```python
from build123d import *

# Parameters (mm, degrees)
SKETCH1_W            = 35
SKETCH1_H            = 30
SKETCH1_R            = 2.1
BOSS_EXTRUDE1_DEPTH  = 5
SKETCH2_W            = 30
SKETCH2_H            = 17
BOSS_EXTRUDE2_DEPTH  = 5
BOSS_EXTRUDE3_START  = -28
BOSS_EXTRUDE3_DEPTH  = 37
CUT_EXTRUDE1_REACH   = 66.542
CUT_EXTRUDE1_START   = -4.5
SKETCH5_W            = 36
SKETCH5_H            = 12.013565991
SKETCH6_W            = 2.1
SKETCH6_H            = 35.25
CUT_EXTRUDE2_DEPTH   = 5
SKETCH7_R            = 2.1
CUT_EXTRUDE3_DEPTH   = 17
SKETCH8_W            = 1.9
SKETCH8_H            = 19
SKETCH8_W_2          = 2.4
BOSS_EXTRUDE4_DEPTH  = 11
SKETCH9_W            = 9.9
SKETCH9_H            = 8
SKETCH9_W_2          = 7.5
BOSS_EXTRUDE5_DEPTH  = 5
BOSS_EXTRUDE6_DEPTH  = 2
BOSS_EXTRUDE7_START  = -13
SKETCH12_R           = 3.3
SKETCH12_R_2         = 2.1
BOSS_EXTRUDE7_DEPTH  = 1
BOSS_EXTRUDE8_START  = -23
SKETCH12_2_R         = 3.3
SKETCH12_2_R_2       = 2.1
BOSS_EXTRUDE8_DEPTH  = 1
SKETCH13_W           = 21.9
SKETCH13_H           = 19
BOSS_EXTRUDE9_DEPTH  = 2
SKETCH14_W           = 1.9
SKETCH14_H           = 19
BOSS_EXTRUDE10_DEPTH = 11
SKETCH15_W           = 21.9
SKETCH15_H           = 19
BOSS_EXTRUDE11_DEPTH = 2
CUT_EXTRUDE4_START   = -36
SKETCH16_R           = 2.1
CUT_EXTRUDE4_DEPTH   = 36
BOSS_EXTRUDE12_START = -2
SKETCH17_R           = 3.3
SKETCH17_R_2         = 2.1
BOSS_EXTRUDE12_DEPTH = 1
BOSS_EXTRUDE13_START = -12
SKETCH17_2_R         = 3.3
SKETCH17_2_R_2       = 2.1
BOSS_EXTRUDE13_DEPTH = 1
CUT_EXTRUDE5_REACH   = 74.341
SKETCH19_R           = 4.5
CUT_EXTRUDE6_REACH   = 69.181
SKETCH20_R           = 1.75
SKETCH21_R           = 1.6
CUT_EXTRUDE7_DEPTH   = 95.781405877


with BuildPart() as part:
    # Sketch1 → Boss-Extrude1 (new body)
    with BuildSketch(Plane(origin=(0, 0, 0), x_dir=(1, 0, 0), z_dir=(0, 1, 0))):
        Rectangle(SKETCH1_W, SKETCH1_H)
        with Locations(Location((12, 9, 0), (0, 0, 270))):
            Circle(SKETCH1_R, mode=Mode.SUBTRACT)
        with Locations(Location((12, -9, 0), (0, 0, 90))):
            Circle(SKETCH1_R, mode=Mode.SUBTRACT)
        with Locations(Location((-12, -9, 0), (0, 0, 270))):
            Circle(SKETCH1_R, mode=Mode.SUBTRACT)
        with Locations(Location((-12, 9, 0), (0, 0, 90))):
            Circle(SKETCH1_R, mode=Mode.SUBTRACT)
    extrude(amount=BOSS_EXTRUDE1_DEPTH)

    # Sketch2 → Boss-Extrude2 (add)
    with BuildSketch(Plane.ZY.offset(17.5)):
        with Locations((0, -3.5)):
            Rectangle(SKETCH2_W, SKETCH2_H)
    extrude(amount=BOSS_EXTRUDE2_DEPTH)

    # Sketch3 → Boss-Extrude3 (add)
    with BuildSketch(Plane(origin=(17.5, 0, 0), x_dir=(0, 0, -1), z_dir=(1, 0, 0)).offset(BOSS_EXTRUDE3_START)):
        with BuildLine():
            Line((-41, 0), (41, 0))
            Line((41, 0), (41, -12))
            Line((41, -12), (37.43, -12))
            Line((37.43, -12), (37.43, -18))
            Line((37.43, -18), (35.03, -18))
            Line((35.03, -18), (35.03, -12))
            Line((35.03, -12), (35.03, -10.095119046))
            ThreePointArc((35.03, -10.095119046), (34.83, -1.9), (34.63, -10.095119046))
            Line((34.63, -10.095119046), (34.63, -12))
            Line((34.63, -12), (34.63, -18))
            Line((34.63, -18), (32.23, -18))
            Line((32.23, -18), (32.23, -12))
            Line((32.23, -12), (-32.23, -12))
            Line((-32.23, -12), (-32.23, -18))
            Line((-32.23, -18), (-34.63, -18))
            Line((-34.63, -18), (-34.63, -12))
            Line((-34.63, -12), (-34.63, -10.095119046))
            ThreePointArc((-34.63, -10.095119046), (-34.83, -1.9), (-35.03, -10.095119046))
            Line((-35.03, -10.095119046), (-35.03, -12))
            Line((-35.03, -12), (-35.03, -18))
            Line((-35.03, -18), (-37.43, -18))
            Line((-37.43, -18), (-37.43, -12))
            Line((-37.43, -12), (-41, -12))
            Line((-41, -12), (-41, 0))
        make_face()
    extrude(amount=-BOSS_EXTRUDE3_DEPTH)

    # Sketch5 → Cut-Extrude1 (cut, up to next)
    with BuildSketch(Plane.ZY.offset(22.5).offset(CUT_EXTRUDE1_START), mode=Mode.PRIVATE) as cut_extrude1_sk1:
        with Locations((0, -5.993217004)):
            Rectangle(SKETCH5_W, SKETCH5_H)
    cut_extrude1_tool1 = extrude(cut_extrude1_sk1.sketch, amount=-CUT_EXTRUDE1_REACH, mode=Mode.PRIVATE) & part.part
    add(cut_extrude1_tool1.solids().sort_by_distance((-18, -5.993217, 0))[0], mode=Mode.SUBTRACT)

    # Sketch6 → Cut-Extrude2 (cut)
    with BuildSketch(Plane(origin=(0, 5, 0), x_dir=(1, 0, 0), z_dir=(0, 1, 0))):
        with Locations((-21.45, -2.625)):
            Rectangle(SKETCH6_W, SKETCH6_H)
    extrude(amount=-CUT_EXTRUDE2_DEPTH, mode=Mode.SUBTRACT)

    # Sketch7 → Cut-Extrude3 (cut)
    with BuildSketch(Plane(origin=(0, 5, 0), x_dir=(1, 0, 0), z_dir=(0, 1, 0))):
        with Locations(Location((-29.9, -20.25, 0), (0, 0, 270))):
            Circle(SKETCH7_R)
        with Locations(Location((-41.9, 20.25, 0), (0, 0, 270))):
            Circle(SKETCH7_R)
    extrude(amount=-CUT_EXTRUDE3_DEPTH, mode=Mode.SUBTRACT)

    # Sketch8 → Boss-Extrude4 (add)
    with BuildSketch(Plane(origin=(0, 0, 0), x_dir=(1, 0, 0), z_dir=(0, 1, 0))):
        with BuildLine():
            Line((-47.5, 10.25), (-34.9, 10.25))
            ThreePointArc((-34.9, 10.25), (-32.778679656, 11.128679656), (-31.9, 13.25))
            Line((-31.9, 13.25), (-31.9, 26.051552427))
            Line((-31.9, 26.051552427), (-30.3, 26.051552427))
            Line((-30.3, 26.051552427), (-30.3, 11.65))
            ThreePointArc((-30.3, 11.65), (-31.178679656, 9.528679656), (-33.3, 8.65))
            Line((-33.3, 8.65), (-47.5, 8.65))
            Line((-47.5, 8.65), (-47.5, 10.25))
        make_face()
        with Locations((-18.95, -20.25)):
            Rectangle(SKETCH8_W, SKETCH8_H)
        with Locations((-38.7, -20.25)):
            Rectangle(SKETCH8_W_2, SKETCH8_H)
    extrude(amount=BOSS_EXTRUDE4_DEPTH)

    # Sketch9 → Boss-Extrude5 (add)
    with BuildSketch(Plane(origin=(0, 0, 0), x_dir=(1, 0, 0), z_dir=(0, 1, 0))):
        with Locations((-15.45, 19)):
            Rectangle(SKETCH9_W, SKETCH9_H)
        with Locations((-14.25, -19)):
            Rectangle(SKETCH9_W_2, SKETCH9_H)
    extrude(amount=BOSS_EXTRUDE5_DEPTH)

    # Sketch10 → Boss-Extrude6 (add)
    with BuildSketch(Plane(origin=(0, 11, 0), x_dir=(1, 0, 0), z_dir=(0, 1, 0))):
        with BuildLine():
            Line((-30.3, 26.051552427), (-47.5, 26.051552427))
            Line((-47.5, 26.051552427), (-47.5, 8.65))
            Line((-47.5, 8.65), (-33.3, 8.65))
            ThreePointArc((-33.3, 8.65), (-31.178679656, 9.528679656), (-30.3, 11.65))
            Line((-30.3, 11.65), (-30.3, 26.051552427))
        make_face()
    extrude(amount=BOSS_EXTRUDE6_DEPTH)

    # Sketch12 → Boss-Extrude7 (add)
    with BuildSketch(Plane.XZ.offset(12).offset(BOSS_EXTRUDE7_START)):
        with Locations(Location((-41.9, -20.25, 0), (0, 0, 270))):
            Circle(SKETCH12_R)
        with Locations(Location((-41.9, -20.25, 0), (0, 0, 90))):
            Circle(SKETCH12_R_2, mode=Mode.SUBTRACT)
    extrude(amount=BOSS_EXTRUDE7_DEPTH)

    # Sketch12<2> → Boss-Extrude8 (add)
    with BuildSketch(Plane.XZ.offset(12).offset(BOSS_EXTRUDE8_START)):
        with Locations(Location((-41.9, -20.25, 0), (0, 0, 270))):
            Circle(SKETCH12_2_R)
        with Locations(Location((-41.9, -20.25, 0), (0, 0, 90))):
            Circle(SKETCH12_2_R_2, mode=Mode.SUBTRACT)
    extrude(amount=BOSS_EXTRUDE8_DEPTH)

    # Sketch13 → Boss-Extrude9 (add)
    with BuildSketch(Plane(origin=(0, 11, 0), x_dir=(1, 0, 0), z_dir=(0, 1, 0))):
        with Locations((-28.95, -20.25)):
            Rectangle(SKETCH13_W, SKETCH13_H)
    extrude(amount=-BOSS_EXTRUDE9_DEPTH)

    # Sketch14 → Boss-Extrude10 (add)
    with BuildSketch(Plane(origin=(0, 11, 0), x_dir=(1, 0, 0), z_dir=(0, 1, 0))):
        with Locations((-18.95, -20.25)):
            Rectangle(SKETCH14_W, SKETCH14_H)
    extrude(amount=BOSS_EXTRUDE10_DEPTH)

    # Sketch15 → Boss-Extrude11 (add)
    with BuildSketch(Plane(origin=(0, 22, 0), x_dir=(1, 0, 0), z_dir=(0, 1, 0))):
        with Locations((-28.95, -20.25)):
            Rectangle(SKETCH15_W, SKETCH15_H)
    extrude(amount=BOSS_EXTRUDE11_DEPTH)

    # Sketch16 → Cut-Extrude4 (cut)
    with BuildSketch(Plane.XZ.offset(12).offset(CUT_EXTRUDE4_START)):
        with Locations(Location((-29.9, 20.25, 0), (0, 0, 90))):
            Circle(SKETCH16_R)
        with Locations(Location((-41.9, -20.25, 0), (0, 0, 90))):
            Circle(SKETCH16_R)
    extrude(amount=CUT_EXTRUDE4_DEPTH, mode=Mode.SUBTRACT)

    # Sketch17 → Boss-Extrude12 (add)
    with BuildSketch(Plane(origin=(0, 24, 0), x_dir=(1, 0, 0), z_dir=(0, 1, 0)).offset(BOSS_EXTRUDE12_START)):
        with Locations(Location((-29.9, -20.25, 0), (0, 0, 270))):
            Circle(SKETCH17_R)
        with Locations(Location((-29.9, -20.25, 0), (0, 0, 270))):
            Circle(SKETCH17_R_2, mode=Mode.SUBTRACT)
    extrude(amount=-BOSS_EXTRUDE12_DEPTH)

    # Sketch17<2> → Boss-Extrude13 (add)
    with BuildSketch(Plane(origin=(0, 24, 0), x_dir=(1, 0, 0), z_dir=(0, 1, 0)).offset(BOSS_EXTRUDE13_START)):
        with Locations(Location((-29.9, -20.25, 0), (0, 0, 270))):
            Circle(SKETCH17_2_R)
        with Locations(Location((-29.9, -20.25, 0), (0, 0, 270))):
            Circle(SKETCH17_2_R_2, mode=Mode.SUBTRACT)
    extrude(amount=-BOSS_EXTRUDE13_DEPTH)

    # Sketch19 → Cut-Extrude5 (cut, up to next)
    with BuildSketch(Plane.XZ.offset(12), mode=Mode.PRIVATE) as cut_extrude5_sk1:
        with Locations(Location((-29.9, 20.25, 0), (0, 0, 270))):
            Circle(SKETCH19_R)
    cut_extrude5_tool1 = extrude(cut_extrude5_sk1.sketch, amount=-CUT_EXTRUDE5_REACH, mode=Mode.PRIVATE) & part.part
    add(cut_extrude5_tool1.solids().sort_by_distance((-29.9, -12, 20.25))[0], mode=Mode.SUBTRACT)

    # Sketch20 → Cut-Extrude6 (cut, up to next)
    with BuildSketch(Plane(origin=(0, 0, 0), x_dir=(1, 0, 0), z_dir=(0, 1, 0)), mode=Mode.PRIVATE) as cut_extrude6_sk1:
        with Locations(Location((-34.5, 4.15, 0), (0, 0, 270))):
            Circle(SKETCH20_R)
    cut_extrude6_tool1 = extrude(cut_extrude6_sk1.sketch, amount=-CUT_EXTRUDE6_REACH, mode=Mode.PRIVATE) & part.part
    # Sketch20 → Cut-Extrude6 (cut, up to next)
    with BuildSketch(Plane(origin=(0, 0, 0), x_dir=(1, 0, 0), z_dir=(0, 1, 0)), mode=Mode.PRIVATE) as cut_extrude6_sk2:
        with Locations(Location((-44.5, -17.85, 0), (0, 0, 270))):
            Circle(SKETCH20_R)
    cut_extrude6_tool2 = extrude(cut_extrude6_sk2.sketch, amount=-CUT_EXTRUDE6_REACH, mode=Mode.PRIVATE) & part.part
    add(cut_extrude6_tool1.solids().sort_by_distance((-34.5, 0, -4.15))[0], mode=Mode.SUBTRACT)
    add(cut_extrude6_tool2.solids().sort_by_distance((-44.5, 0, 17.85))[0], mode=Mode.SUBTRACT)

    # Sketch21 → Cut-Extrude7 (cut, through all)
    with BuildSketch(Plane(origin=(0, 0, -37.43), x_dir=(-1, 0, 0), z_dir=(0, 0, -1))):
        with Locations((19.5, -15)):
            Circle(SKETCH21_R)
        with Locations((38.5, -15)):
            Circle(SKETCH21_R)
    extrude(amount=-CUT_EXTRUDE7_DEPTH, mode=Mode.SUBTRACT)


solid = part.part
```
Check sheet for the modelled part. Datum: model origin and axes. Units: mm. A direction names the side the tool comes from. Give positions to 0.01 mm unless a question says otherwise; leave off trailing zeros. Write each loop counter-clockwise with the first axis right and the second up, starting at its lowest first coordinate (ties: lowest second). Pieces come first, ordered by that corner, then holes.
Item 1: Cross-section at C-C (z = -4.15). Enter the section's corners in (x, y).
Item 2: Gauge pin test, flat ends, axial feed: pin 1 (7.5 mm diameter, centred on x = -43.5, z = -19.5, fed in from -Y); pin 2 (5.5 mm diameter, centred on x = -39.5, y = 8, fed in from -Z); pin 3 (5 mm diameter, centred on x = -9.5, z = 10.5, fed in from +Y); pin 4 (5 mm diameter, centred on y = 15.5, z = 7, fed in from -X). Record the tip position at first contact, or that the pin passes through.
Item 3: Access from +Z, -Z, +X, -X, +Y, -Y to the whole of each face (thin tool, end or side, straight path). Record for faces 4 (the face through (-39.9, 23, 20)), 5 (the face through (-30, 22, 24)), 6 (the face through (-29, -12, 39)), 7 (the face through (-14, -6, 18)), 8 (the face through (-29, -14, 34.63)).
Item 4: Cross-section at D-D (z = -28). Enter the section's corners in (x, y).
Item 5: Cross-section at B-B (x = 12). Enter the section's corners in (y, z), and give its area (3 significant figures).
Item 6: Scan lines: L1, parallel to Z at x = 12, y = 1.7; L2, parallel to X at y = 2, z = 9; L3, parallel to Z at x = -39, y = -6. Record each from-to range of solid material in increasing order.
Item 7: Cross-section at A-A (y = -6). Enter the section's corners in (x, z).
Item 8: Draft check along Y on faces 1 (the face through (-14, 0, -17)), 2 (the face through (-39.1, 0.5, -22)), 3 (the face through (-43.982, 11.521, -20.523)). Enter one of: released by +Y, released by -Y, zero draft, split by the parting line, or undercut.
Report:
1. outline: (-47.5, -12) - (-36.25, -12) - (-36.25, 0) - (-47.5, 0) - close; (-32.75, -12) - (-18, -12) - (-18, 0.01) - (17.5, 0.01) - (17.5, 5) - (-20.4, 5) - (-20.4, 0) - (-32.75, 0) - close
2. pin 1: stops at y = -12
2. pin 2: stops at z = -23.51
2. pin 3: stops at y = 5
2. pin 4: passes through
3. face 4: +Z, -Z, -X, +Y
3. face 5: none
3. face 6: +Z, +X, -X, -Y
3. face 7: +X, -Y
3. face 8: +X, -X, -Y
4. outline: (-47.5, -12) - (-10.5, -12) - (-10.5, 0) - (-47.5, 0) - close
5. outline: (0.01, -15) - (5, -15) - (5, -11.1) - (0.01, -11.1) - close; (0.01, -6.9) - (5, -6.9) - (5, 6.9) - (0.01, 6.9) - close; (0.01, 11.1) - (5, 11.1) - (5, 15) - (0.01, 15) - close
5. area: 108 mm2
6. L1: z = -15 to -11.1, -6.9 to 6.9, 11.1 to 15
6. L2: x = -20.4 to -14.1, -9.9 to 9.9, 14.1 to 17.5
6. L3: z = -41 to -38.93, -30.73 to 30.73, 38.93 to 41
7. outline: (-47.5, -41) - (-10.5, -41) - (-10.5, -38.93) - (-47.5, -38.93) - close; (-47.5, -30.73) - (-10.5, -30.73) - (-10.5, -18) - (-18, -18) - (-18, 18) - (-10.5, 18) - (-10.5, 30.73) - (-47.5, 30.73) - close; (-47.5, 38.93) - (-10.5, 38.93) - (-10.5, 41) - (-47.5, 41) - close; hole circle Ø3.5 at (-44.5, 17.85); hole circle Ø4.2 at (-41.9, -20.25); hole circle Ø3.5 at (-34.5, -4.15); hole circle Ø9 at (-29.9, 20.25)
8. face 1: released by -Y
8. face 2: undercut
8. face 3: zero draft
